from build123d import *

# Parameters (mm, degrees)
SHELL1_T = -2.286


with BuildPart() as part:
    # Sketch1 → Revolve1 (revolve)
    with BuildSketch(Plane(origin=(0, 0, 0), x_dir=(0, 0, -1), z_dir=(1, 0, 0)), mode=Mode.PRIVATE) as revolve1_sk:
        with BuildLine():
            Line((113.538, 0), (-113.538, 0))
            Line((-113.538, 0), (-113.538, 10.16))
            Line((-113.538, 10.16), (-103.378, 10.16))
            ThreePointArc((-103.378, 10.16), (-94.01066843, 21.251164674), (-80.09851547, 25.4))
            Line((-80.09851547, 25.4), (80.09851547, 25.4))
            ThreePointArc((80.09851547, 25.4), (94.01066843, 21.251164674), (103.378, 10.16))
            Line((103.378, 10.16), (113.538, 10.16))
            Line((113.538, 10.16), (113.538, 0))
        make_face()
    revolve(revolve1_sk.sketch.rotate(Axis((0, 0, -113.538), (0, 0, 1)), 90), axis=Axis((0, 0, -113.538), (0, 0, 1)))

    # Shell1
    shell1_openings = [part.faces().sort_by_distance(p)[0] for p in [
        (0, 0, 113.538),
        (0, 0, -113.538),
    ]]
    offset(amount=SHELL1_T, openings=shell1_openings, kind=Kind.INTERSECTION)


solid = part.part
The listing builds one solid part. Answer for the finished solid, in the listing's coordinates (mm). A direction names the side the tool comes from. Give positions to 0.01 mm unless a question says otherwise; leave off trailing zeros. Write each loop counter-clockwise with the first axis right and the second up, starting at its lowest first coordinate (ties: lowest second). Pieces come first, ordered by that corner, then holes. Notation, with made-up numbers: (63, -40) -> (92, -40) arc R12 cw to (92, -29) -> close; hole circle Ø9 at (86.25, -37.75). An arc over 180 degrees is marked (long way). Use a Markdown table: item, result.
(1) Section B-B, the plane y = -18.5 is taken. Determine the outline of the cut face in (x, z).
Return value:
| item | result |
|---|---|
| outline | (-17.4, -80.1) arc R17.4 ccw to (17.4, -80.1) -> (17.4, 80.1) arc R17.4 ccw to (-17.4, 80.1) -> close; hole (-13.86, -80.1) arc R13.86 ccw to (13.86, -80.1) -> (13.86, 80.1) arc R13.86 ccw to (-13.86, 80.1) -> close |
(2) Section C-C, the plane x = 21 is taken. Determine the outline of the cut face in (y, z), then the cut area to 3 significant figures.
Return value:
| item | result |
|---|---|
| outline | (-14.29, -80.1) arc R14.29 ccw to (14.29, -80.1) -> (14.29, 80.1) arc R14.29 ccw to (-14.29, 80.1) -> close; hole (-9.66, -80.1) arc R9.66 ccw to (9.66, -80.1) -> (9.66, 80.1) arc R9.66 ccw to (-9.66, 80.1) -> close |
| area | 1,830 mm2 |
(3) Section A-A, the plane x = 0 is taken. Determine the outline of the cut face in (y, z).
Return value:
| item | result |
|---|---|
| outline | (-25.4, -80.1) arc R25.4 ccw to (-10.16, -103.38) -> (-10.16, -113.54) -> (-7.87, -113.54) -> (-7.87, -101.83) arc R23.11 cw to (-23.11, -80.1) -> (-23.11, 80.1) arc R23.11 cw to (-7.87, 101.83) -> (-7.87, 113.54) -> (-10.16, 113.54) -> (-10.16, 103.38) arc R25.4 ccw to (-25.4, 80.1) -> close; (7.87, -113.54) -> (10.16, -113.54) -> (10.16, -103.38) arc R25.4 ccw to (25.4, -80.1) -> (25.4, 80.1) arc R25.4 ccw to (10.16, 103.38) -> (10.16, 113.54) -> (7.87, 113.54) -> (7.87, 101.83) arc R23.11 cw to (23.11, 80.1) -> (23.11, -80.1) arc R23.11 cw to (7.87, -101.83) -> close |
(4) Section D-D, the plane z = -59 is taken. Determine the outline of the cut face in (x, y).
Return value:
| item | result |
|---|---|
| outline | circle Ø50.8 at (0, 0); hole circle Ø46.23 at (0, 0) |
(5) For faces 1 (the cylindrical face through (20.157, 15.456, -1.121)), 2 (the cylindrical face through (1.323, -10.074, -108.529)), determine the directions among +Z, -Z, +X, -X, +Y, -Y from which every point of the face is accessible in a straight line to the end or side of a thin tool.
Return value:
| item | result |
|---|---|
| face 1 | +Z, -Z |
| face 2 | -Z |
(6) Find the intervals of material crossed by probe 1 along Y at (x, z) = (0, -105); probe 2 along Y at (x, z) = (-0.5, -59); probe 3 along Z at (x, y) = (-3, -9.5), in increasing order. Write a range as from..to.
Return value:
| item | result |
|---|---|
| probe 1 | -10.16..-7.87, 7.87..10.16 |
| probe 2 | -25.4..-23.11, 23.11..25.4 |
| probe 3 | -113.54..-100.96, 100.96..113.54 |
(7) Determine the mould class of faces 3 (the cylindrical face through (3.009, -22.917, -1.121)), 4 (the flat face through (-3, 7.5, -113.538)), 5 (the cylindrical face through (1.323, -10.074, 108.387)) for opening direction X: released by +X, released by -X, zero draft, split by the parting line, or undercut.
Return value:
| item | result |
|---|---|
| face 3 | undercut |
| face 4 | zero draft |
| face 5 | split by the parting line |
(8) Flat-ended cylindrical pins translate along their axes: P1, Ø12.5, axis at x = 0, y = 0, coming from the -Z side; P2, Ø6, axis at x = 2, z = -72, coming from the -Y side; P3, Ø8, axis at x = 17.5, y = 4, coming from the +Z side; P4, Ø2, axis at y = 19.5, z = -39, coming from the -X side. Find the tip coordinate at first contact, or state that the pin passes through.
Return value:
| item | result |
|---|---|
| P1 | through |
| P2 | y = -25.4 |
| P3 | z = 101.32 |
| P4 | x = -17.4 |
